Read the model definition and answer for the solid it produces. Units are mm, in the model's axes. A direction names the side the tool comes from. Give positions to 0.01 mm unless a question says otherwise; leave off trailing zeros. Order: outer loops, then holes, each group sorted by start corner. A loop starts at its lowest first (then second) coordinate and runs counter-clockwise, first axis right, second up. Notation, with made-up numbers: (18.5, 39) - (59.5, 39) arc R21 cw to (59.5, 69) - close; hole circle Ø7 at (-22.5, 87.25). An arc over 180 degrees is marked (long way). Return JSON: item names as keys, results as strings.
```python
from build123d import *

# Parameters (mm, degrees)
F0_W      = 101.6
F0_H      = 50.8
F1_DEPTH  = 12.7
F2_R      = 25.39999
F3_R      = 12.7
F4_DEPTH  = 12.701
F5_W      = 38.1
F5_H      = 12.7
F6_DEPTH  = 44.45
F7_R      = 19.04999
F8_W      = 38.1
F8_H      = 12.7
F9_DEPTH  = 44.45
F10_R     = 19.04999
F11_R     = 9.525
F12_DEPTH = 50.801


# Not quite as in the source:
# - a fillet or chamfer is up to 0.001 mm smaller than in the source, because OpenCascade refuses the exact size


with BuildPart() as f1:
    # F0 (on Top) → F1 (new body)
    with BuildSketch(Plane.XY):
        with Locations((2.7364386797, -9.4244979978)):
            Rectangle(F0_W, F0_H)
    extrude(amount=F1_DEPTH)

    # F2 (radius 25.4 in the source; OpenCascade refuses exactly that, so slightly less here)
    f2_edges = [f1.edges().sort_by_distance(p)[0] for p in [
        (-48.063561, 15.975502, 6.35),
        (-48.063561, -34.824498, 6.35),
    ]]
    fillet(f2_edges, radius=F2_R)

    # F3 (on face) → F4 (cut, through all)
    with BuildSketch(Plane.XY.offset(12.7)):
        with Locations((-22.6635613203, -9.4244979978)):
            Circle(F3_R)
    extrude(amount=-F4_DEPTH, mode=Mode.SUBTRACT)

    # F5 (on face) → F6 (join)
    with BuildSketch(Plane.XY.offset(12.7)):
        with Locations((34.4864386797, -28.4744979978)):
            Rectangle(F5_W, F5_H)
    extrude(amount=F6_DEPTH)

    # F7 (radius 19.05 in the source; OpenCascade refuses exactly that, so slightly less here)
    f7_edges = [f1.edges().sort_by_distance(p)[0] for p in [
        (15.436439, -28.474498, 57.15),
        (53.536439, -28.474498, 57.15),
    ]]
    fillet(f7_edges, radius=F7_R)

    # F8 (on face) → F9 (join)
    with BuildSketch(Plane.XY.offset(12.7)):
        with Locations((34.4864386797, 9.6255020022)):
            Rectangle(F8_W, F8_H)
    extrude(amount=F9_DEPTH)

    # F10 (radius 19.05 in the source; OpenCascade refuses exactly that, so slightly less here)
    f10_edges = [f1.edges().sort_by_distance(p)[0] for p in [
        (15.436439, 9.625502, 57.15),
        (53.536439, 9.625502, 57.15),
    ]]
    fillet(f10_edges, radius=F10_R)

    # F11 (on face) → F12 (cut, through all)
    with BuildSketch(Plane.XZ.offset(34.8244979978)):
        with Locations((34.3096069992, 38.1)):
            Circle(F11_R)
    extrude(amount=-F12_DEPTH, mode=Mode.SUBTRACT)


solid = f1.part
```
Q1. Determine the mould class of faces 1 (the flat face through (15.436, -29, 25)), 2 (the cylindrical face through (-16.8, -20.69, 6.44)), 3 (the flat face through (23, -34.824, 22)), 4 (the cylindrical face through (33.07, -28.563, 47.544)) for opening direction X: released by +X, released by -X, zero draft, split by the parting line, or undercut.
Values:
{"face 1": "released by -X", "face 2": "undercut", "face 3": "zero draft", "face 4": "undercut"}
Q2. Consider L1, parallel to Y at x = 42.5, z = 52; L2, parallel to Z at x = -38, y = -10; L3, parallel to X at y = -28, z = 23. Determine where each line is inside the solid, lowest interval first.
Values:
{"L1": "y = -34.82 to -22.12, 3.28 to 15.98", "L2": "z = 0 to 12.7", "L3": "x = 15.44 to 53.54"}
Q3. A cutting plane is placed at B-B (y = -19). Write down the section's boundary in (x, z).
Values:
{"outline": "(-46.19, 0) - (-31.01, 0) - (-31.01, 12.7) - (-46.19, 12.7) - close; (-14.32, 0) - (53.54, 0) - (53.54, 12.7) - (-14.32, 12.7) - close"}
Q4. A cutting plane is placed at C-C (x = -19.5). Write down the section's boundary in (y, z), and give its area (3 significant figures).
Values:
{"outline": "(-34.82, 0) - (-21.72, 0) - (-21.72, 12.7) - (-34.82, 12.7) - close; (2.88, 0) - (15.98, 0) - (15.98, 12.7) - (2.88, 12.7) - close", "area": "333 mm²"}
Q5. Given pin 1 (3 mm diameter, centred on x = 16, y = -3, fed in from +Z); pin 2 (3 mm diameter, centred on y = -21.5, z = 28.5, fed in from -X); pin 3 (11.5 mm diameter, centred on x = 34.31, z = 38.1, fed in from -Y), each flat-ended and moving along its own axis, determine where each tip first touches the part or whether it passes through.
Values:
{"pin 1": "stops at z = 12.7", "pin 2": "stops at x = 15.44", "pin 3": "passes through"}
Q6. For faces 5 (the cylindrical face through (47.808, 9.714, 51.718)), 6 (the flat face through (2, -9, 12.7)), 7 (the flat face through (34, -22.124, 25)), 8 (the flat face through (15.436, 10, 25)), determine the directions among +Z, -Z, +X, -X, +Y, -Y from which every point of the face is accessible in a straight line to the end or side of a thin tool.
Values:
{"face 5": "+Z, +X, +Y, -Y", "face 6": "+Z, -X", "face 7": "+Z, +X, -X", "face 8": "+Z, -X, +Y, -Y"}
